from build123d import *

# Parameters (mm, degrees)
ESBO_O1_R                = 11.75
ESBO_O1_R_2              = 1.6
RESSALTO_EXTRUS_O1_DEPTH = 6
FILETE3_R                = 5


with BuildPart() as part:
    # Esboço1 → Ressalto-extrusão1 (new body)
    with BuildSketch(Plane.XY):
        with BuildLine():
            Line((-15.491933385, -4), (-29, -4))
            Line((-29, -4), (-6.831996166, -14.468027799))
            ThreePointArc((-6.831996166, -14.468027799), (-12.328193669, -10.198805854), (-15.491933385, -4))
        make_face()
        with BuildLine():
            Line((-29, -4), (-15.491933385, -4))
            ThreePointArc((-15.491933385, -4), (0, -16), (15.491933385, -4))
            Line((15.491933385, -4), (29, -4))
            Line((29, -4), (29, 4))
            Line((29, 4), (15.491933385, 4))
            ThreePointArc((15.491933385, 4), (0, 16), (-15.491933385, 4))
            Line((-15.491933385, 4), (-29, 4))
            Line((-29, 4), (-29, -4))
        make_face()
        Circle(ESBO_O1_R, mode=Mode.SUBTRACT)
        with Locations((-25, 0)):
            Circle(ESBO_O1_R_2, mode=Mode.SUBTRACT)
        with Locations((25, 0)):
            Circle(ESBO_O1_R_2, mode=Mode.SUBTRACT)
        with BuildLine():
            Line((-6.831996166, 14.468027799), (-29, 4))
            Line((-29, 4), (-15.491933385, 4))
            ThreePointArc((-15.491933385, 4), (-12.328193669, 10.198805854), (-6.831996166, 14.468027799))
        make_face()
        with BuildLine():
            Line((29, 4), (6.831996166, 14.468027799))
            ThreePointArc((6.831996166, 14.468027799), (12.328193669, 10.198805854), (15.491933385, 4))
            Line((15.491933385, 4), (29, 4))
        make_face()
        with BuildLine():
            ThreePointArc((15.491933385, -4), (12.328193669, -10.198805854), (6.831996166, -14.468027799))
            Line((6.831996166, -14.468027799), (29, -4))
            Line((29, -4), (15.491933385, -4))
        make_face()
    extrude(amount=RESSALTO_EXTRUS_O1_DEPTH)

    # Filete3
    filete3_edges = [part.edges().sort_by_distance(p)[0] for p in [
        (29, 4, 3),
        (29, -4, 3),
        (-29, -4, 3),
        (-29, 4, 3),
    ]]
    fillet(filete3_edges, radius=FILETE3_R)


solid = part.part
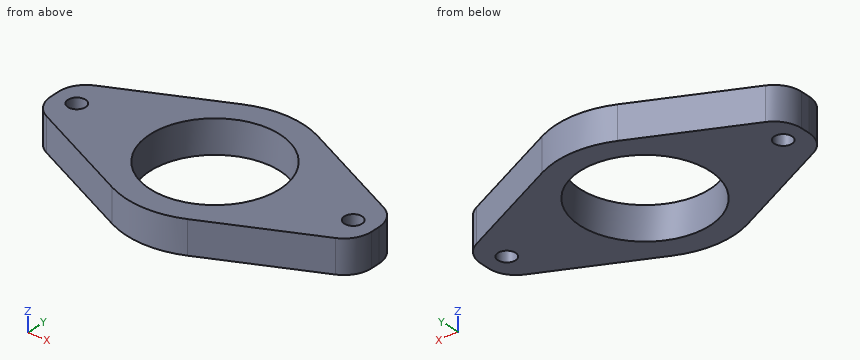
Check sheet for the modelled part. Datum: model origin and axes. Units: mm. Give positions to 0.01 mm unless a question says otherwise; leave off trailing zeros. Write each loop counter-clockwise with the first axis right and the second up, starting at its lowest first coordinate (ties: lowest second). Pieces come first, ordered by that corner, then holes. Notation, with made-up numbers: (28, -28) -> (64, -28) arc R20 ccw to (64, -8) -> close; hole circle Ø2 at (14, -40). An arc over 180 degrees is marked (long way). One line per item, written item: value. Start each with the question number.
Item 1: Section check C-C on y = 0. Record the cut outline in (x, z).
Item 2: Section check A-A on z = 4.4. Record the cut outline in (x, y) (3 decimals).
Item 3: Section check B-B on x = 0. Record the cut outline in (y, z).
Item 4: Section check D-D on y = 4.5. Record the cut outline in (x, z).
Item 5: Gauge pin test, flat ends, axial feed: pin 1 (1.5 mm diameter, centred on x = 17.5, z = 1.5, fed in from -Y); pin 2 (3 mm diameter, centred on y = 4.5, z = 1.5, fed in from -X); pin 3 (2 mm diameter, centred on y = 4.5, z = 3.5, fed in from +X). Record the tip position at first contact, or that the pin passes through.
Item 6: Material ranges on probe 1 along Y at (x, z) = (-0.5, 3.4); probe 2 along X at (y, z) = (-2, 3.1); probe 3 along X at (y, z) = (-5, 5), recorded low to high. Write a range as from..to.
Results list:
1. outline: (-29, 0) -> (-26.6, 0) -> (-26.6, 6) -> (-29, 6) -> close; (-23.4, 0) -> (-11.75, 0) -> (-11.75, 6) -> (-23.4, 6) -> close; (11.75, 0) -> (23.4, 0) -> (23.4, 6) -> (11.75, 6) -> close; (26.6, 0) -> (29, 0) -> (29, 6) -> (26.6, 6) -> close
2. outline: (-29, -0.832) arc R5 ccw to (-26.135, -5.353) -> (-6.832, -14.468) arc R16 ccw to (6.832, -14.468) -> (26.135, -5.353) arc R5 ccw to (29, -0.832) -> (29, 0.832) arc R5 ccw to (26.135, 5.353) -> (6.832, 14.468) arc R16 ccw to (-6.832, 14.468) -> (-26.135, 5.353) arc R5 ccw to (-29, 0.832) -> close; hole circle Ø3.2 at (-25, 0); hole circle Ø23.5 at (0, 0); hole circle Ø3.2 at (25, 0)
3. outline: (-16, 0) -> (-11.75, 0) -> (-11.75, 6) -> (-16, 6) -> close; (11.75, 0) -> (16, 0) -> (16, 6) -> (11.75, 6) -> close
4. outline: (-27.4, 0) -> (-10.85, 0) -> (-10.85, 6) -> (-27.4, 6) -> close; (10.85, 0) -> (27.4, 0) -> (27.4, 6) -> (10.85, 6) -> close
5. pin 1: y = -9.78
5. pin 2: x = -28.51
5. pin 3: x = 28.23
6. probe 1: -15.99..-11.74, 11.74..15.99
6. probe 2: -28.86..-11.58, 11.58..28.86
6. probe 3: -26.76..-10.63, 10.63..26.76
